Geometry: see drawing. Coordinates: mm, zero at the bounding-box minimum. Coordinates: 2 decimals unless noted, no trailing zeros. Order: outer loops, then holes, each group sorted by start corner. A loop starts at its lowest first (then second) coordinate and runs counter-clockwise, first axis right, second up.
Item 1: Contact query for flat-ended pins moving along their axis: P1, Ø7.5, axis at x = 61.5, y = 47.5, coming from the +Z side; P2, Ø2.5, axis at x = 91, z = 1, coming from the +Y side; P3, Ø4, axis at y = 18.5, z = 4.5, coming from the -X side; P4, Ø1, axis at x = 34, y = 27, coming from the +Z side (3 decimals). Output: stop coordinate, or through.
Item 2: Mould query, pull axis Z, two halves, no side actions, for the marked faces 1, 2 and 3. Classes: released by +Z, released by -Z, zero draft, split by the parting line, or undercut.
Item 3: Section A-A on x = 50. Return the cut outline in (y, z).
Item 4: Section C-C on z = 4.5. Return the cut outline in (x, y).
Item 5: Ray query, line 1 (Z direction, x = 55.5, y = 58.5); line 2 (Z direction, x = 41, y = 33); line 3 (Y direction, x = 47.5, z = 9.5). Return the intervals inside material, ascending.
Item 6: Section B-B on y = 20. Return the cut outline in (x, z), then the cut area to 3 significant figures.
Item 7: Section D-D on x = 75. Return the cut outline in (y, z), then the cut area to 3 significant figures.
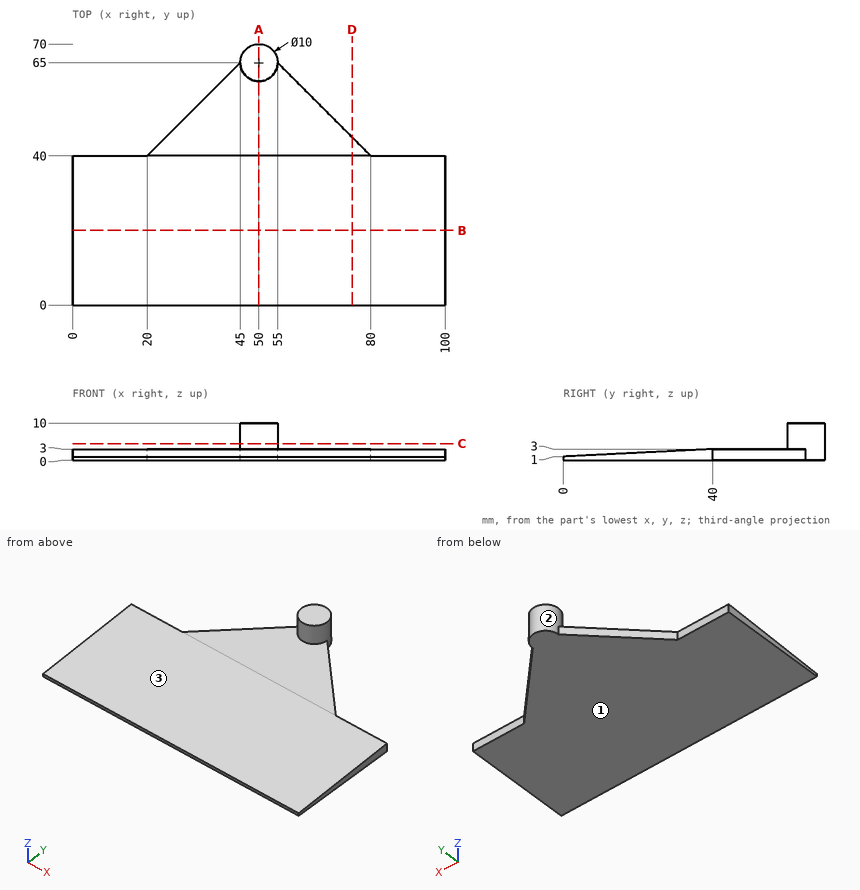
Answer list:
1. P1: stops at z = 3
1. P2: stops at y = 40
1. P3: passes through
1. P4: stops at z = 2.375
2. face 1: released by -Z
2. face 2: zero draft
2. face 3: released by +Z
3. outline: (0, 0) - (70, 0) - (70, 10) - (60, 10) - (60, 3) - (40, 3) - (0, 1) - close
4. outline: circle Ø10 at (50, 65)
5. line 1: z = 0 to 3
5. line 2: z = 0 to 2.65
5. line 3: y = 60.67 to 69.33
6. outline: (0, 0) - (100, 0) - (100, 2) - (0, 2) - close
6. area: 200 mm2
7. outline: (0, 0) - (45, 0) - (45, 3) - (40, 3) - (0, 1) - close
7. area: 95.0 mm2
